from build123d import *

# Parameters (mm, degrees)
F1_DEPTH = 25.4


with BuildPart() as f1:
    # F0 (on Top) → F1 (new body)
    with BuildSketch(Plane.XY):
        Polygon((-46.93308, 0), (0, -19.440318), (46.93308, 0), (0, 113.306479), align=None)
        Polygon((21.53308, 5.959682), (-25.4, 5.959682), (-1.93346, 36.541872), align=None, mode=Mode.SUBTRACT)
    extrude(amount=F1_DEPTH)


solid = f1.part
Geometry check sheet. Reference: the model listing, model coordinates, mm. A direction names the side the tool comes from. Coordinates: 2 decimals unless noted, no trailing zeros. Order: outer loops, then holes, each group sorted by start corner. A loop starts at its lowest first (then second) coordinate and runs counter-clockwise, first axis right, second up. Notation, with made-up numbers: (-34.5, 36.5) -> (0.5, 36.5) arc R8 cw to (0.5, 45.5) -> close; hole circle Ø1 at (-5.75, 88). An arc over 180 degrees is marked (long way). Use a Markdown table: item, result. Add a question column.
1. Go/stop test with flat-tipped pins: pin 1 Ø6 at (x, z) = (-28.5, 9) entering from -Y; pin 2 Ø12 at (x, y) = (1, 10) entering from -Z; pin 3 Ø4 at (y, z) = (77, 7) entering from -X; pin 4 Ø10 at (x, z) = (25.5, 5) entering from -Y. Record where each tip stops, or that it passes through.
2. Cross-section at D-D (y = 103). Enter the section's corners in (x, z), and give its area (3 significant figures).
3. Cross-section at A-A (z = 10.25). Enter the section's corners in (x, y), and give its area (3 significant figures).
4. Cross-section at B-B (y = 33). Enter the section's corners in (x, z), and give its area (3 significant figures).
5. Mould release check, pull along X, two halves, no side actions. Record for faces 3 (the face through (-13.83, 21.04, 12.52)), 4 (the face through (23.795, 55.86, 12.522)), 5 (the face through (10, 33, 25.4)), 6 (the face through (9.64, 21.46, 12.52)): pulls with the +X half, pulls with the -X half, needs draft (parallel to the pull), parting line crosses it, or undercut.
6. Set-up check for faces 1 (the face through (-2, 5.96, 13)), 2 (the face through (10, 33, 0)): record each of +Z, -Z, +X, -X, +Y, -Y from which the full face is reachable in a straight line by a thin tool's end or side.
7. Material ranges on L1, parallel to X at y = 11, z = 6.25; L2, parallel to Y at x = 15, z = 7.5; L3, parallel to X at y = 30.5, z = 3, recorded low to high.
8. Cross-section at C-C (x = -4). Enter the section's corners in (y, z).
Filled sheet:
| question | item | result |
|---|---|---|
| 1 | pin 1 | y = -8.88 |
| 1 | pin 2 | z = 0 |
| 1 | pin 3 | x = -15.87 |
| 1 | pin 4 | y = -10.95 |
| 2 | outline | (-4.27, 0) -> (4.27, 0) -> (4.27, 25.4) -> (-4.27, 25.4) -> close |
| 2 | area | 217 mm2 |
| 3 | outline | (-46.93, 0) -> (0, -19.44) -> (46.93, 0) -> (0, 113.31) -> close; hole (-25.4, 5.96) -> (21.53, 5.96) -> (-1.93, 36.54) -> close |
| 3 | area | 5,510 mm2 |
| 4 | outline | (-33.26, 0) -> (-4.65, 0) -> (-4.65, 25.4) -> (-33.26, 25.4) -> close; (0.78, 0) -> (33.26, 0) -> (33.26, 25.4) -> (0.78, 25.4) -> close |
| 4 | area | 1,550 mm2 |
| 5 | face 3 | undercut |
| 5 | face 4 | pulls with the +X half |
| 5 | face 5 | needs draft |
| 5 | face 6 | undercut |
| 6 | face 1 | +Z, -Z |
| 6 | face 2 | -Z, +X, -X, +Y, -Y |
| 7 | L1 | -42.38 to -21.53, 17.67 to 42.38 |
| 7 | L2 | -13.23 to 5.96, 14.47 to 77.09 |
| 7 | L3 | -34.3 to -6.57, 2.7 to 34.3 |
| 8 | outline | (-17.78, 0) -> (5.96, 0) -> (5.96, 25.4) -> (-17.78, 25.4) -> close; (33.85, 0) -> (103.65, 0) -> (103.65, 25.4) -> (33.85, 25.4) -> close |
